Model file for the job. Use its own axes, mm. Face numbers are marked on the shaded views. A direction names the side the tool comes from. Round coordinates to 2 decimals unless told otherwise and drop trailing zeros. Write each loop counter-clockwise with the first axis right and the second up, starting at its lowest first coordinate (ties: lowest second). Pieces come first, ordered by that corner, then holes. Notation, with made-up numbers: (59.25, -8) - (83.25, -8) arc R25 cw to (83.25, 16) - close; hole circle Ø2 at (84, -30). An arc over 180 degrees is marked (long way). One line per item, written item: value.
Autodesk Inventor part; units mm, degrees
ref_plane "YZ Plane" through (0, 0, 0) normal (1, 0, 0) x (0, 1, 0)
ref_plane "XZ Plane" through (0, 0, 0) normal (0, 1, 0) x (-1, 0, 0)
ref_plane "XY Plane" through (0, 0, 0) normal (0, 0, 1) x (1, 0, 0)
sketch "Sketch1" plane through (0, 0, 0) normal (0, 0, 1) x (1, 0, 0)
  circle A0 centre (0, 0) radius 29.0893
  dimension "d0" = 58.1787
extrude "Extrusion1" add sketch "Sketch1" along normal blind 10.1905
sketch "Sketch2" plane through (0, 0, 10.1905) normal (0, 0, 1) x (1, 0, 0)
  line L0 (0, 7.239) -> (6.2692, 3.6195)
  line L1 (6.2692, 3.6195) -> (6.2692, -3.6195)
  line L2 (6.2692, -3.6195) -> (0, -7.239)
  line L3 (0, -7.239) -> (-6.2692, -3.6195)
  line L4 (-6.2692, -3.6195) -> (-6.2692, 3.6195)
  line L5 (-6.2692, 3.6195) -> (0, 7.239)
  point P0 (0, 0)
  point P1 (0, 0)
  point P2 (0, 0)
  dimension "d5" = 14.478
extrude "Extrusion2" cut sketch "Sketch2" against normal blind 10.1905
properties part number "large gear hex"
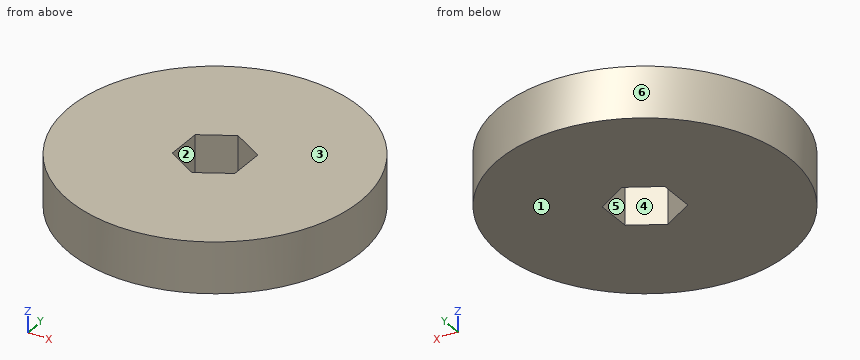
1. Drop flat-ended pins along their axis: pin 1 (5 mm diameter, centred on x = -6, z = 5.5, fed in from +Y); pin 2 (3 mm diameter, centred on y = 7, z = 8.5, fed in from +X); pin 3 (1 mm diameter, centred on x = -0.5, z = 4.5, fed in from +Y). Give the stop position or say it passes through.
Report:
pin 1: y = 28.88
pin 2: x = 28.56
pin 3: y = 29.09
2. Band-saw the part on B-B on z = 3. Write the cut outline in (x, y).
Report:
outline: circle Ø58.18 at (0, 0); hole (-6.27, -3.62) - (0, -7.24) - (6.27, -3.62) - (6.27, 3.62) - (0, 7.24) - (-6.27, 3.62) - close
3. Tool access for the marked faces 1 and 2: list every direction of +Z, -Z, +X, -X, +Y, -Y with a clear straight run to the whole face (end or side of a thin tool).
Report:
face 1: -Z, +X, -X, +Y, -Y
face 2: +Z, -Z
4. Band-saw the part on A-A on y = 0. Write the cut outline in (x, z), plus the area to 3 significant figures.
Report:
outline: (-29.09, 0) - (-6.27, 0) - (-6.27, 10.19) - (-29.09, 10.19) - close; (6.27, 0) - (29.09, 0) - (29.09, 10.19) - (6.27, 10.19) - close
area: 465 mm²
5. Mould opens along Y. For the marked faces 3, 4, 5 and 6 say: released by +Y, released by -Y, zero draft, split by the parting line, or undercut.
Report:
face 3: zero draft
face 4: undercut
face 5: undercut
face 6: split by the parting line
6. Band-saw the part on D-D on x = -7.5. Write the cut outline in (y, z), plus the area to 3 significant figures.
Report:
outline: (-28.11, 0) - (28.11, 0) - (28.11, 10.19) - (-28.11, 10.19) - close
area: 573 mm²
7. Wall check: probe 1 along Y at (x, z) = (0, 2); probe 2 along Y at (x, z) = (5.5, 8.75); probe 3 along X at (y, z) = (-3, 3). Give the ranges that are in metal, low to high. Write a range as [from, to].
Report:
probe 1: [-29.09, -7.24], [7.24, 29.09]
probe 2: [-28.56, -4.06], [4.06, 28.56]
probe 3: [-28.93, -6.27], [6.27, 28.93]
8. Band-saw the part on C-C on x = 3. Write the cut outline in (y, z).
Report:
outline: (-28.93, 0) - (-5.51, 0) - (-5.51, 10.19) - (-28.93, 10.19) - close; (5.51, 0) - (28.93, 0) - (28.93, 10.19) - (5.51, 10.19) - close
